The drawing under review shows one solid part. Ordinate dimensions are in mm from its lowest x, y, z. A direction names the side the tool comes from. Round coordinates to 2 decimals unless told otherwise and drop trailing zeros. Order: outer loops, then holes, each group sorted by start corner. A loop starts at its lowest first (then second) coordinate and runs counter-clockwise, first axis right, second up. Notation, with made-up numbers: M -39.75,31.25 L -6.75,31.25 A29 cw -6.75,60.25 Z; hole C 54.25,26.25 d11. An arc over 180 degrees is marked long. Write item = value, one per line. Start each with the question number.
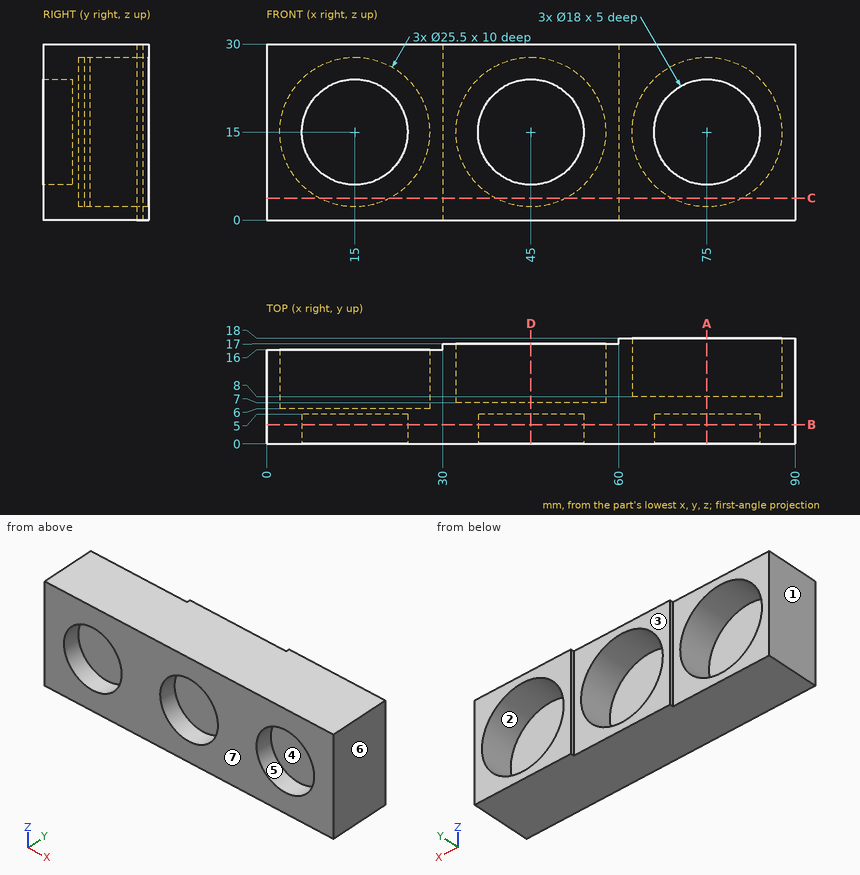
(1) Consider section A-A, the plane x = 75. Write out the cut boundary in (y, z).
(2) Draft analysis for pull direction X (two halves, no side actions). For the marked faces 5, 6 and 7, state which applies: pulls with the +X half, pulls with the -X half, needs draft (parallel to the pull), parting line crosses it, or undercut.
(3) Insertion check: pin 1 (0.5 mm diameter, centred on y = 17.5, z = 13, fed in from -X); pin 2 (7.5 mm diameter, centred on x = 76.5, z = 12, fed in from +Y); pin 3 (1 mm diameter, centred on x = 12, z = 6, fed in from -Y); pin 4 (9 mm diameter, centred on x = 51.5, z = 11.5, fed in from +Y). Each pin has a flat end and moves straight along its axis. Give the tip position at first contact, or say it passes through.
(4) For line 1 along X through (y, z) = (2.4, 15); line 2 along X through (y, z) = (8.5, 15); line 3 along Y through (x, z) = (42.5, 23.25), list the stretches that pass through material, from the lowest coordinate up. Write a range as [from, to].
(5) Consider section D-D, the plane x = 45. Write out the cut boundary in (y, z), then the cut area to 3 significant figures.
(6) Consider section B-B, the plane y = 3.25. Write out the cut boundary in (x, z), then the cut area to 3 significant figures.
(7) Consider section C-C, the plane z = 3.75. Write out the cut boundary in (x, y).
(8) For the marked faces 1, 2, 3 and 4, list the 3-axis set-ups (+Z, -Z, +X, -X, +Y, -Y) from which the entire face can be reached by the end or side of a thin tool; tool diameter is ignored.
Completed:
q1.outline = M 0,0 L 18,0 L 18,2.25 L 8,2.25 L 8,27.75 L 18,27.75 L 18,30 L 0,30 L 0,24 L 5,24 L 5,6 L 0,6 Z
q2.face_5 = undercut
q2.face_6 = pulls with the +X half
q2.face_7 = needs draft
q3.pin_1 = 60
q3.pin_2 = 8
q3.pin_3 = 0
q3.pin_4 = 7
q4.line_1 = [0, 6], [24, 36], [54, 66], [84, 90]
q4.line_2 = [0, 2.25], [27.75, 32.25], [57.75, 62.25], [87.75, 90]
q4.line_3 = [5, 7]
q5.outline = M 0,0 L 17,0 L 17,2.25 L 7,2.25 L 7,27.75 L 17,27.75 L 17,30 L 0,30 L 0,24 L 5,24 L 5,6 L 0,6 Z
q5.area = 165 mm2
q6.outline = M 0,0 L 90,0 L 90,30 L 0,30 Z; hole C 15,15 d18; hole C 45,15 d18; hole C 75,15 d18
q6.area = 1,940 mm2
q7.outline = M 0,0 L 90,0 L 90,18 L 81,18 L 81,8 L 69,8 L 69,18 L 60,18 L 60,17 L 51,17 L 51,7 L 39,7 L 39,17 L 30,17 L 30,16 L 21,16 L 21,6 L 9,6 L 9,16 L 0,16 Z
q8.face_1 = +Z, -Z, -X, +Y, -Y
q8.face_2 = +Y
q8.face_3 = +Z, -Z, -X, +Y
q8.face_4 = -Y
